Geometry: final body of the model. Coordinates: model frame, mm. A direction names the side the tool comes from. Round coordinates to 2 decimals unless told otherwise and drop trailing zeros. Loops run counter-clockwise (first coordinate to the right, second up) from the corner with the lowest first, then second, coordinate; pieces in that order, holes last. Notation, with made-up numbers: M 62.5,76 L 118.5,76 A25 ccw 118.5,89 Z; hole C 33.25,-9 d9. An arc over 180 degrees is marked long. Answer as a JSON object with one key per item and string values.
```python
from build123d import *

# Parameters (mm, degrees)
SKETCH1_R                      = 11.5
BOSS_EXTRUDE1_DEPTH            = 60
CUT_EXTRUDE1_REACH             = 167.294
SKETCH2_R                      = 3
CUT_EXTRUDE1_DIRECTION_2_DEPTH = 166.294105853
SKETCH3_W                      = 11
SKETCH3_H                      = 10
CUT_EXTRUDE2_DEPTH             = 5
SKETCH5_R                      = 11
BOSS_EXTRUDE2_DEPTH            = 60
SKETCH5_12_R                   = 11
CUT_EXTRUDE7_DEPTH             = 6
SKETCH5_13_R                   = 5
CUT_EXTRUDE8_DEPTH             = 189.480626049
CUT_EXTRUDE9_START             = -6
SKETCH5_14_R                   = 1
CUT_EXTRUDE9_DEPTH             = 6


with BuildPart() as part:
    # Sketch1 → Boss-Extrude1 (new body)
    with BuildSketch(Plane(origin=(0, 0, 0), x_dir=(1, 0, 0), z_dir=(0, 1, 0))):
        with BuildLine():
            Line((17.257858547, 56.070568137), (17.257858547, 46.070568137))
            Line((17.257858547, 46.070568137), (34.625468063, 46.070568137))
            ThreePointArc((34.625468063, 46.070568137), (99.590834225, 44.570568137), (34.625468063, 43.070568137))
            Line((34.625468063, 43.070568137), (17.257858547, 43.070568137))
            Line((17.257858547, 43.070568137), (17.257858547, 33.070568137))
            Line((17.257858547, 33.070568137), (28.257858547, 33.070568137))
            ThreePointArc((28.257858547, 33.070568137), (86.245043845, 8.88631035), (98.136101416, 70.579054926))
            ThreePointArc((98.136101416, 70.579054926), (96.534674627, 82.125537677), (107.090834225, 87.070568137))
            ThreePointArc((107.090834225, 87.070568137), (124.590834225, 104.570568137), (107.090834225, 122.070568137))
            Line((107.090834225, 122.070568137), (27.090834225, 122.070568137))
            ThreePointArc((27.090834225, 122.070568137), (9.590834225, 104.570568137), (27.090834225, 87.070568137))
            ThreePointArc((27.090834225, 87.070568137), (37.646993822, 82.125537677), (36.045567034, 70.579054926))
            ThreePointArc((36.045567034, 70.579054926), (31.406576437, 63.724777757), (28.257858547, 56.070568137))
            Line((28.257858547, 56.070568137), (17.257858547, 56.070568137))
        make_face()
        with Locations(Location((27.090834225, 104.570568137, 0), (0, 0, 270))):
            Circle(SKETCH1_R, mode=Mode.SUBTRACT)
        with Locations(Location((107.090834225, 104.570568137, 0), (0, 0, 270))):
            Circle(SKETCH1_R, mode=Mode.SUBTRACT)
    extrude(amount=BOSS_EXTRUDE1_DEPTH)

    # Cut-Extrude1: up to this face of the body (flat: up to its plane)
    cut_extrude1_end = Plane(part.part.faces().sort_by_distance((22.757858547, 30, -56.070568137))[0])
    # Sketch2 → Cut-Extrude1 (cut, up to the picked face)
    with BuildSketch(Plane(origin=(-1.111756956, 0, -33.070568137), x_dir=(1, 0, 0), z_dir=(0, 0, 1)), mode=Mode.PRIVATE) as cut_extrude1_sk1:
        with Locations(Location((23.869615503, 30, 0), (0, 0, 180))):
            Circle(SKETCH2_R)
    cut_extrude1_tool1 = split(extrude(cut_extrude1_sk1.sketch, amount=-CUT_EXTRUDE1_REACH, mode=Mode.PRIVATE), bisect_by=cut_extrude1_end, keep=Keep.BOTH, mode=Mode.PRIVATE)
    # Sketch2 → Cut-Extrude1 (cut, up to the picked face)
    with BuildSketch(Plane(origin=(-1.111756956, 0, -33.070568137), x_dir=(1, 0, 0), z_dir=(0, 0, 1)), mode=Mode.PRIVATE) as cut_extrude1_sk2:
        with Locations(Location((23.869615503, 50, 0), (0, 0, 180))):
            Circle(SKETCH2_R)
    cut_extrude1_tool2 = split(extrude(cut_extrude1_sk2.sketch, amount=-CUT_EXTRUDE1_REACH, mode=Mode.PRIVATE), bisect_by=cut_extrude1_end, keep=Keep.BOTH, mode=Mode.PRIVATE)
    # Sketch2 → Cut-Extrude1 (cut, up to the picked face)
    with BuildSketch(Plane(origin=(-1.111756956, 0, -33.070568137), x_dir=(1, 0, 0), z_dir=(0, 0, 1)), mode=Mode.PRIVATE) as cut_extrude1_sk3:
        with Locations(Location((23.869615503, 10, 0), (0, 0, 180))):
            Circle(SKETCH2_R)
    cut_extrude1_tool3 = split(extrude(cut_extrude1_sk3.sketch, amount=-CUT_EXTRUDE1_REACH, mode=Mode.PRIVATE), bisect_by=cut_extrude1_end, keep=Keep.BOTH, mode=Mode.PRIVATE)
    add(cut_extrude1_tool1.solids().sort_by(Axis((22.757859, 30, -33.070568), (0, 0, -1)))[0], mode=Mode.SUBTRACT)
    add(cut_extrude1_tool2.solids().sort_by(Axis((22.757859, 50, -33.070568), (0, 0, -1)))[0], mode=Mode.SUBTRACT)
    add(cut_extrude1_tool3.solids().sort_by(Axis((22.757859, 10, -33.070568), (0, 0, -1)))[0], mode=Mode.SUBTRACT)

    # Sketch2 → Cut-Extrude1 direction 2 (cut)
    with BuildSketch(Plane(origin=(-1.111756956, 0, -33.070568137), x_dir=(1, 0, 0), z_dir=(0, 0, 1))):
        with Locations(Location((23.869615503, 30, 0), (0, 0, 180))):
            Circle(SKETCH2_R)
        with Locations(Location((23.869615503, 50, 0), (0, 0, 180))):
            Circle(SKETCH2_R)
        with Locations(Location((23.869615503, 10, 0), (0, 0, 180))):
            Circle(SKETCH2_R)
    extrude(amount=CUT_EXTRUDE1_DIRECTION_2_DEPTH, mode=Mode.SUBTRACT)

    # Sketch3 → Cut-Extrude2 (cut)
    with BuildSketch(Plane(origin=(0, 0, -56.070568137), x_dir=(-1, 0, 0), z_dir=(0, 0, -1))):
        with Locations((-22.757858547, 50)):
            Rectangle(SKETCH3_W, SKETCH3_H)
        with Locations((-22.757858547, 30)):
            Rectangle(SKETCH3_W, SKETCH3_H)
        with Locations((-22.757858547, 10)):
            Rectangle(SKETCH3_W, SKETCH3_H)
    extrude(amount=-CUT_EXTRUDE2_DEPTH, mode=Mode.SUBTRACT)

    # Sketch5 → Boss-Extrude2 (add)
    with BuildSketch(Plane(origin=(0, 60, 0), x_dir=(1, 0, 0), z_dir=(0, 1, 0))):
        with Locations((67.090834225, 117.070568137)):
            Circle(SKETCH5_R)
    extrude(amount=-BOSS_EXTRUDE2_DEPTH)

    # Sketch5<12> → Cut-Extrude7 (cut)
    with BuildSketch(Plane(origin=(0, 60, 0), x_dir=(1, 0, 0), z_dir=(0, 1, 0))):
        with Locations((67.090834225, 117.070568137)):
            Circle(SKETCH5_12_R)
    extrude(amount=-CUT_EXTRUDE7_DEPTH, mode=Mode.SUBTRACT)

    # Sketch5<13> → Cut-Extrude8 (cut, through all)
    with BuildSketch(Plane(origin=(0, 60, 0), x_dir=(1, 0, 0), z_dir=(0, 1, 0))):
        with Locations(Location((67.090834225, 117.070568137, 0), (0, 0, 270))):
            Circle(SKETCH5_13_R)
    extrude(amount=-CUT_EXTRUDE8_DEPTH, mode=Mode.SUBTRACT)

    # Sketch5<14> → Cut-Extrude9 (cut)
    with BuildSketch(Plane(origin=(0, 60, 0), x_dir=(1, 0, 0), z_dir=(0, 1, 0)).offset(CUT_EXTRUDE9_START)):
        with Locations(Location((67.090834225, 125.070568137, 0), (0, 0, 270))):
            Circle(SKETCH5_14_R)
        with Locations(Location((75.090834225, 117.070568137, 0), (0, 0, 270))):
            Circle(SKETCH5_14_R)
        with Locations(Location((67.090834225, 109.070568137, 0), (0, 0, 270))):
            Circle(SKETCH5_14_R)
        with Locations(Location((59.090834225, 117.070568137, 0), (0, 0, 270))):
            Circle(SKETCH5_14_R)
    extrude(amount=-CUT_EXTRUDE9_DEPTH, mode=Mode.SUBTRACT)


solid = part.part
```
1) Line query: probe 1 along Y at (x, z) = (27, -53.5); probe 2 along X at (y, z) = (10, -39); probe 3 along Z at (x, y) = (37, 5). Output: solid intervals per line, ascending.
Geometry results:
{"probe 1": "0 to 5, 15 to 25, 35 to 45, 55 to 60", "probe 2": "17.26 to 19.76, 25.76 to 35.07, 99.11 to 107.21", "probe 3": "-122.07 to -110.41, -98.73 to -83.16, -71.72 to -56.85, -32.29 to -17.46"}
2) Cut plane C-C on y = 19. Return the cut outline in (x, z) (3 decimals).
Geometry results:
{"outline": "M 17.258,-56.071 L 28.258,-56.071 A40.5 ccw 36.046,-70.579 A9.822 cw 27.091,-87.071 A17.5 ccw 27.091,-122.071 L 57.293,-122.071 A11 ccw 76.889,-122.071 L 107.091,-122.071 A17.5 ccw 107.091,-87.071 A9.822 cw 98.136,-70.579 A40.5 ccw long 28.258,-33.071 L 17.258,-33.071 L 17.258,-43.071 L 34.625,-43.071 A32.5 cw long 34.625,-46.071 L 17.258,-46.071 Z; hole C 27.091,-104.571 d23; hole C 67.091,-117.071 d10; hole C 107.091,-104.571 d23"}
3) Cut plane A-A on y = 50. Count the separate pieces of the cut face and the enclosed holes in it, and give its area (3 significant figures).
Geometry results:
{"separate pieces": "3", "enclosed holes": "7", "area": "5,140 mm2"}
4) Cut plane B-B on y = 30. Return the cut outline in (x, z) (3 decimals).
Geometry results:
{"outline": "M 17.258,-51.071 L 19.758,-51.071 L 19.758,-46.071 L 17.258,-46.071 Z; M 17.258,-43.071 L 19.758,-43.071 L 19.758,-33.071 L 17.258,-33.071 Z; M 25.758,-51.071 L 28.258,-51.071 L 28.258,-56.071 A40.5 ccw 36.046,-70.579 A9.822 cw 27.091,-87.071 A17.5 ccw 27.091,-122.071 L 57.293,-122.071 A11 ccw 76.889,-122.071 L 107.091,-122.071 A17.5 ccw 107.091,-87.071 A9.822 cw 98.136,-70.579 A40.5 ccw long 28.258,-33.071 L 25.758,-33.071 L 25.758,-43.071 L 34.625,-43.071 A32.5 cw long 34.625,-46.071 L 25.758,-46.071 Z; hole C 27.091,-104.571 d23; hole C 67.091,-117.071 d10; hole C 107.091,-104.571 d23"}
5) First-contact query: pin 1 (8 mm diameter, centred on x = 25, y = 51, fed in from -Z); pin 2 (1.5 mm diameter, centred on y = 19, z = -103.5, fed in from +X); pin 3 (4 mm diameter, centred on y = 7, z = -77, fed in from -X). Flat tips, straight axial feed; report the tip coordinate or a pass-through.
Geometry results:
{"pin 1": "z = -122.07", "pin 2": "x = 124.59", "pin 3": "x = 38.53"}
6) Pull-direction query (Y, two-part tool) for faces 1 (the face through (23, 57, -56.071)), 2 (the face through (69, 54, -112)), 3 (the face through (24.969, 47.972, -48.536)), 4 (the face through (28.258, 50, -54)); classes: +Y half, -Y half, draft (parallel to the pull), parting line (faces both ways), or undercut.
Geometry results:
{"face 1": "draft", "face 2": "+Y half", "face 3": "undercut", "face 4": "undercut"}
7) Set-up query: faces 5 (the face through (17.258, 30, -50)), 6 (the face through (25.755, 9.868, -48.536)), 7 (the face through (23, 55, -54)), 8 (the face through (26, 30, -46.071)). Return all of +Z, -Z, +X, -X, +Y, -Y with unobstructed straight access to the full face (end or side cutting, diameter ignored); none if empty.
Geometry results:
{"face 5": "+Z, -X, +Y, -Y", "face 6": "+Z", "face 7": "-X", "face 8": "-X, +Y, -Y"}
